from build123d import *

# Parameters (mm, degrees)
SKETCH1_W                    = 215.9
SKETCH1_H                    = 152.4
BOSS_EXTRUDE1_DEPTH          = 88.9
F_5_8_0_625_DIAMETER_HOLE1_D = 15.875
SKETCH9_W                    = 127
SKETCH9_H                    = 63.5
CUT_EXTRUDE1_DEPTH           = 279.822129681


with BuildPart() as part:
    # Sketch1 → Boss-Extrude1 (new body)
    with BuildSketch(Plane(origin=(0, 0, 0), x_dir=(1, 0, 0), z_dir=(0, 1, 0))):
        with Locations((-107.95, 76.2)):
            Rectangle(SKETCH1_W, SKETCH1_H)
    extrude(amount=BOSS_EXTRUDE1_DEPTH)

    # 5/8 (0.625) Diameter Hole1 (through all)
    with Locations(Plane.XY):
        with Locations((-190.5, 25.4), (-25.4, 25.4)):
            Hole(F_5_8_0_625_DIAMETER_HOLE1_D / 2)

    # Sketch9 → Cut-Extrude1 (cut, through all)
    with BuildSketch(Plane(origin=(0, 0, 0), x_dir=(0, 0, -1), z_dir=(1, 0, 0))):
        with Locations((76.2, 44.45)):
            Rectangle(SKETCH9_W, SKETCH9_H)
    extrude(amount=-CUT_EXTRUDE1_DEPTH, mode=Mode.SUBTRACT)


solid = part.part
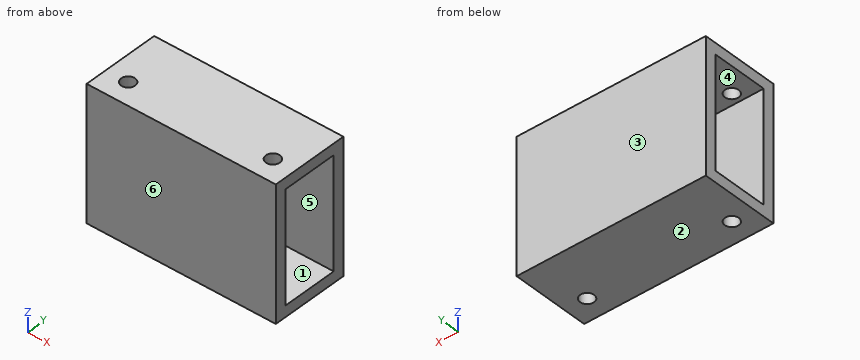
Can you work these out from the model? Positions are in its coordinate system, mm. Face numbers are marked on the shaded views. A direction names the side the tool comes from. Coordinates: 2 decimals unless noted, no trailing zeros. Loops run counter-clockwise (first coordinate to the right, second up) from the corner with the lowest first, then second, coordinate; pieces in that order, holes last. Notation, with made-up numbers: M 14.25,62 L 59.25,62 A13 ccw 59.25,85 Z; hole C 33,7.5 d6. An arc over 180 degrees is marked long. Return JSON: item names as keys, results as strings. Group by question number.
Item 1: On a 3-axis mill with a long thin cutter (end or side, diameter ignored), from which of +Z, -Z, +X, -X, +Y, -Y can I reach the whole of each face in a straight line? I mean the marked faces 1 and 2. Say none if no direction works.
Item 2: Imagine slicing it at B-B (y = 25.4). Please give me the cut outline in (x, z), and give its area (3 significant figures).
Item 3: If I drill on L1, parallel to Y at x = -202, z = -132; L2, parallel to Z at x = -142, y = 43; L3, parallel to X at y = 25, z = -9, over which ranges is the centre line in solid material (lowest first)? Write a range as from..to.
Item 4: Thinking about a two-plate mould opening in Y: for the marked faces 3, 4, 5 and 6, which applies, released by +Y, released by -Y, zero draft, split by the parting line, or undercut?
Item 5: Imagine slicing it at C-C (x = -129). Please give me the cut outline in (y, z), and give its area (3 significant figures).
Item 6: Imagine slicing it at D-D (z = -68.5). Please give me the cut outline in (x, y), and give its area (3 significant figures).
Item 7: I'm going to push a flat-ended pin straight in: pin 1 Ø18.5 at (x, y) = (-190.5, 25.4) entering from -Z. Where does the tip first touch, or does it pass through?
Item 8: Imagine slicing it at A-A (y = 71). Please give me the cut outline in (x, z).
Verdict:
{
 "1": {"face 1": "+X, -X", "face 2": "-Z, +X, -X, +Y, -Y"},
 "2": {"outline": "M -215.9,-152.4 L -198.44,-152.4 L -198.44,-139.7 L -215.9,-139.7 Z; M -215.9,-12.7 L -198.44,-12.7 L -198.44,0 L -215.9,0 Z; M -182.56,-152.4 L -33.34,-152.4 L -33.34,-139.7 L -182.56,-139.7 Z; M -182.56,-12.7 L -33.34,-12.7 L -33.34,0 L -182.56,0 Z; M -17.46,-152.4 L 0,-152.4 L 0,-139.7 L -17.46,-139.7 Z; M -17.46,-12.7 L 0,-12.7 L 0,0 L -17.46,0 Z", "area": "4,680 mm^2"},
 "3": {"L1": "y = 0..12.7, 76.2..88.9", "L2": "z = -152.4..-139.7, -12.7..0", "L3": "x = -215.9..-198.43, -182.57..-33.33, -17.47..0"},
 "4": {"face 3": "released by +Y", "face 4": "undercut", "face 5": "undercut", "face 6": "released by -Y"},
 "5": {"outline": "M 0,-152.4 L 88.9,-152.4 L 88.9,0 L 0,0 Z; hole M 12.7,-139.7 L 76.2,-139.7 L 76.2,-12.7 L 12.7,-12.7 Z", "area": "5,480 mm^2"},
 "6": {"outline": "M -215.9,0 L 0,0 L 0,12.7 L -215.9,12.7 Z; M -215.9,76.2 L 0,76.2 L 0,88.9 L -215.9,88.9 Z", "area": "5,480 mm^2"},
 "7": {"pin 1": "stops at z = -152.4"},
 "8": {"outline": "M -215.9,-152.4 L 0,-152.4 L 0,-139.7 L -215.9,-139.7 Z; M -215.9,-12.7 L 0,-12.7 L 0,0 L -215.9,0 Z"}
}
